Verification items for the finished model (mm, model axes). Face numbers are marked on the shaded views. A direction names the side the tool comes from. Coordinates: 2 decimals unless noted, no trailing zeros. Order: outer loops, then holes, each group sorted by start corner. A loop starts at its lowest first (then second) coordinate and runs counter-clockwise, first axis right, second up. Notation, with made-up numbers: M 20.5,86 L 41.5,86 A17 ccw 41.5,100 Z; hole C 54,43.5 d3. An arc over 180 degrees is marked long. Return JSON: item names as keys, results as strings. Group by question number.
Q1. Section check C-C, the plane y = 16.5. Enter the section's corners in (x, z), then the cut area to 3 significant figures.
Q2. Section check B-B, the plane y = 1. Enter the section's corners in (x, z).
Q3. Access from +Z, -Z, +X, -X, +Y, -Y to the whole of each face (thin tool, end or side, straight path). Record for the marked faces 1, 2 and 3.
Q4. Section check A-A, the plane z = -8.89. Count the separate pieces of the cut face and the enclosed holes in it, then the cut area to 3 significant figures.
Q5. Go/stop test with flat-tipped pins: pin 1 Ø5.5 at (y, z) = (13.5, -9.5) entering from +X; pin 2 Ø2 at (y, z) = (-14.5, -5) entering from -X; pin 3 Ø8 at (x, y) = (-8.73, 0) entering from +Z. Record where each tip stops, or that it passes through.
Q6. Mould release check, pull along X, two halves, no side actions. Record for the marked faces 4, 5 and 6: pulls with the +X half, pulls with the -X half, needs draft (parallel to the pull), parting line crosses it, or undercut.
Q7. Thickness scan on probe 1 along Y at (x, z) = (-49.5, -6.25); probe 2 along Z at (x, y) = (-72.5, 4.5); probe 3 along X at (y, z) = (0.5, -3). Record the ranges inside material, lowest first.
from build123d import *

# Parameters (mm, degrees)
SKETCH1_W           = 93.6625
SKETCH1_H           = 40.64
SKETCH1_R           = 2.4892
BOSS_EXTRUDE1_DEPTH = 17.78
SKETCH6_R           = 3.96875
CUT_EXTRUDE4_DEPTH  = 104.635910312
CUT_EXTRUDE3_DEPTH  = 17.78
FILLET1_R           = 2.54
SKETCH3_R           = 4.064
CUT_EXTRUDE5_DEPTH  = 4.7752
CUT_EXTRUDE6_DEPTH  = 98.141100599


with BuildPart() as part:
    # Sketch1 → Boss-Extrude1 (new body)
    with BuildSketch(Plane.XY):
        with Locations((-46.83125, 0)):
            Rectangle(SKETCH1_W, SKETCH1_H)
        with Locations((-84.93125, 0)):
            Circle(SKETCH1_R, mode=Mode.SUBTRACT)
        with Locations((-8.73125, 0)):
            Circle(SKETCH1_R, mode=Mode.SUBTRACT)
    extrude(amount=-BOSS_EXTRUDE1_DEPTH)

    # Sketch6 → Cut-Extrude4 (cut, through all)
    with BuildSketch(Plane(origin=(0, 20.32, 0), x_dir=(1, 0, 0), z_dir=(0, 1, 0))):
        with Locations(Location((-72.23125, 8.89, 0), (0, 0, 270))):
            Circle(SKETCH6_R)
        with Locations(Location((-21.43125, 8.89, 0), (0, 0, 270))):
            Circle(SKETCH6_R)
    extrude(amount=-CUT_EXTRUDE4_DEPTH, mode=Mode.SUBTRACT)

    # Sketch5 → Cut-Extrude3 (cut)
    with BuildSketch(Plane.XY):
        with BuildLine():
            Line((-93.6625, -20.32), (-93.6625, 20.32))
            Line((-93.6625, 20.32), (-84.93125, 20.32))
            Line((-84.93125, 20.32), (-84.93125, 10.622546022))
            ThreePointArc((-84.93125, 10.622546022), (-85.477262526, 9.049137635), (-86.880552326, 8.152186482))
            ThreePointArc((-86.880552326, 8.152186482), (-93.31325, 0), (-86.880552326, -8.152186482))
            ThreePointArc((-86.880552326, -8.152186482), (-85.477262526, -9.049137635), (-84.93125, -10.622546022))
            Line((-84.93125, -10.622546022), (-84.93125, -20.32))
            Line((-84.93125, -20.32), (-93.6625, -20.32))
        make_face()
        with BuildLine():
            Line((0, -20.32), (0, 20.32))
            Line((0, 20.32), (-8.73125, 20.32))
            Line((-8.73125, 20.32), (-8.73125, 10.622546022))
            ThreePointArc((-8.73125, 10.622546022), (-8.185237474, 9.049137635), (-6.781947674, 8.152186482))
            ThreePointArc((-6.781947674, 8.152186482), (-0.34925, 0), (-6.781947674, -8.152186482))
            ThreePointArc((-6.781947674, -8.152186482), (-8.185237474, -9.049137635), (-8.73125, -10.622546022))
            Line((-8.73125, -10.622546022), (-8.73125, -20.32))
            Line((-8.73125, -20.32), (0, -20.32))
        make_face()
    extrude(amount=-CUT_EXTRUDE3_DEPTH, mode=Mode.SUBTRACT)

    # Fillet1
    fillet1_edges = [part.edges().sort_by_distance(p)[0] for p in [
        (-84.93125, 20.32, -8.89),
        (-84.93125, -20.32, -8.89),
        (-8.73125, 20.32, -8.89),
        (-8.73125, -20.32, -8.89),
    ]]
    fillet(fillet1_edges, radius=FILLET1_R)

    # Sketch3 → Cut-Extrude5 (cut)
    with BuildSketch(Plane.XY):
        with Locations((-84.93125, 0)):
            Circle(SKETCH3_R)
        with Locations((-8.73125, 0)):
            Circle(SKETCH3_R)
    extrude(amount=-CUT_EXTRUDE5_DEPTH, mode=Mode.SUBTRACT)

    # Sketch7 → Cut-Extrude6 (cut, through all)
    with BuildSketch(Plane.XY):
        with BuildLine():
            Line((-59.53125, -15.24), (-34.13125, -15.24))
            ThreePointArc((-34.13125, -15.24), (-32.335198776, -14.496051224), (-31.59125, -12.7))
            Line((-31.59125, -12.7), (-31.59125, 12.7))
            ThreePointArc((-31.59125, 12.7), (-32.335198776, 14.496051224), (-34.13125, 15.24))
            Line((-34.13125, 15.24), (-59.53125, 15.24))
            ThreePointArc((-59.53125, 15.24), (-61.327301224, 14.496051224), (-62.07125, 12.7))
            Line((-62.07125, 12.7), (-62.07125, -12.7))
            ThreePointArc((-62.07125, -12.7), (-61.327301224, -14.496051224), (-59.53125, -15.24))
        make_face()
    extrude(amount=-CUT_EXTRUDE6_DEPTH, mode=Mode.SUBTRACT)


solid = part.part
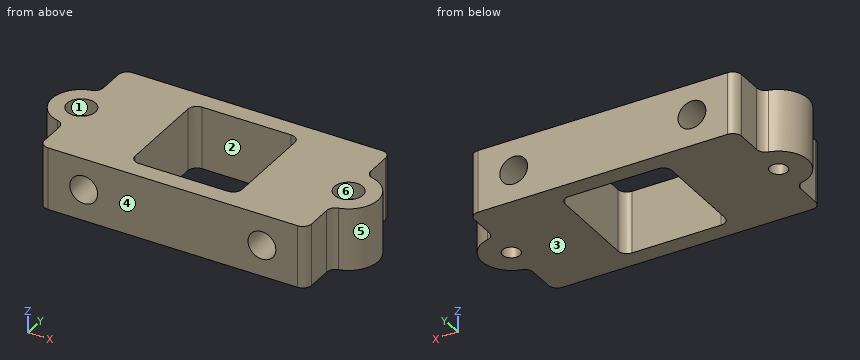
Numbers:
{
 "1": {"outline": "M -84.93,-17.78 L -8.73,-17.78 L -8.73,0 L -84.93,0 Z; hole C -72.23,-8.89 d7.94; hole C -21.43,-8.89 d7.94", "area": "1,260 mm2"},
 "2": {"outline": "M -93.25,-17.78 L -87.21,-17.78 L -87.21,-4.78 L -88.87,-4.78 L -88.87,0 L -93.25,0 Z; M -82.65,-17.78 L -62.07,-17.78 L -62.07,0 L -80.99,0 L -80.99,-4.78 L -82.65,-4.78 Z; M -31.59,-17.78 L -11.01,-17.78 L -11.01,-4.78 L -12.67,-4.78 L -12.67,0 L -31.59,0 Z; M -6.45,-17.78 L -0.41,-17.78 L -0.41,0 L -4.79,0 L -4.79,-4.78 L -6.45,-4.78 Z; hole C -72.23,-8.89 d7.94; hole C -21.43,-8.89 d7.94"},
 "3": {"face 1": "+Z", "face 2": "+Z, -Z", "face 3": "-Z, +X, -X, +Y, -Y"},
 "4": {"separate pieces": "3", "enclosed holes": "3", "area": "1,710 mm2"},
 "5": {"pin 1": "stops at x = -8.73", "pin 2": "stops at x = -84.93", "pin 3": "stops at z = -4.78"},
 "6": {"face 4": "needs draft", "face 5": "pulls with the +X half", "face 6": "undercut"},
 "7": {"probe 1": "y = -20.32 to -15.24, 15.24 to 20.32", "probe 2": "z = -17.78 to -12.85, -4.93 to 0", "probe 3": "x = -93.3 to -88.96, -80.9 to -62.07, -31.59 to -12.76, -4.7 to -0.36"}
}
